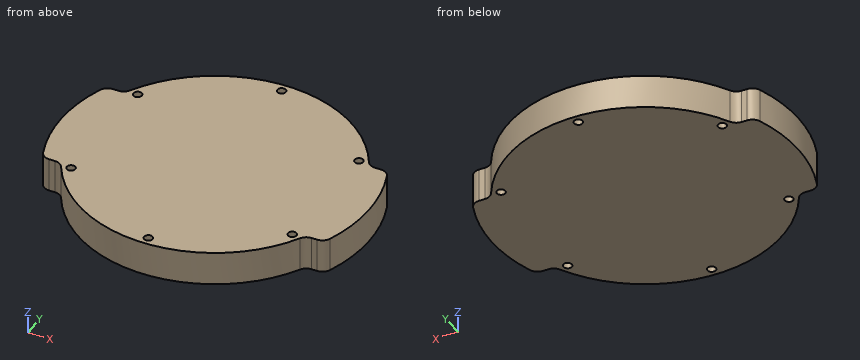
```python
from build123d import *

# Parameters (mm, degrees)
SKETCH_1_R          = 45.3
EXTRUDE_1_DEPTH     = 10
CUT_EXTRUDE_1_DEPTH = 11
FILLET_1_R          = 3
SKETCH_3_R          = 1.25
CUT_EXTRUDE_2_DEPTH = 11


with BuildPart() as part:
    # 草图1 → 凸台-拉伸1 (new body)
    with BuildSketch(Plane.XY):
        Circle(SKETCH_1_R)
    extrude(amount=EXTRUDE_1_DEPTH)

    # 草图2 → 切除-拉伸1 (cut, through all)
    with BuildSketch(Plane.XY.offset(10)):
        with BuildLine():
            Line((-36.056760808, 18), (-41.570301899, 18))
            ThreePointArc((-41.570301899, 18), (0, 45.3), (41.570301899, 18))
            Line((41.570301899, 18), (36.056760808, 18))
            ThreePointArc((36.056760808, 18), (0, 40.3), (-36.056760808, 18))
        make_face()
        with BuildLine():
            Line((-36.056760808, -18), (-41.734622438, -18))
            ThreePointArc((-41.734622438, -18), (0, -45.450838386), (41.734622438, -18))
            Line((41.734622438, -18), (36.056760808, -18))
            ThreePointArc((36.056760808, -18), (0, -40.3), (-36.056760808, -18))
        make_face()
    extrude(amount=-CUT_EXTRUDE_1_DEPTH, mode=Mode.SUBTRACT)

    # 圆角1
    fillet_1_edges = [part.edges().sort_by_distance(p)[0] for p in [
        (36.056760808, 18, 5),
        (-36.056760808, 18, 5),
        (-41.570301899, 18, 5),
        (41.570301899, 18, 5),
        (41.570301899, -18, 5),
        (36.056760808, -18, 5),
        (-41.570301899, -18, 5),
        (-36.056760808, -18, 5),
    ]]
    fillet(fillet_1_edges, radius=FILLET_1_R)

    # 草图3 → 切除-拉伸2 (cut, through all)
    with BuildSketch(Plane.XY.offset(10)):
        with Locations((0, 37.7)):
            Circle(SKETCH_3_R)
        with Locations((32.649157723, 18.85)):
            Circle(SKETCH_3_R)
        with Locations((32.649157723, -18.85)):
            Circle(SKETCH_3_R)
        with Locations((0, -37.7)):
            Circle(SKETCH_3_R)
        with Locations((-32.649157723, -18.85)):
            Circle(SKETCH_3_R)
        with Locations((-32.649157723, 18.85)):
            Circle(SKETCH_3_R)
    extrude(amount=-CUT_EXTRUDE_2_DEPTH, mode=Mode.SUBTRACT)


solid = part.part
```
Geometry check sheet. Reference: the model listing, model coordinates, mm. Give positions to 0.01 mm unless a question says otherwise; leave off trailing zeros. Write each loop counter-clockwise with the first axis right and the second up, starting at its lowest first coordinate (ties: lowest second). Pieces come first, ordered by that corner, then holes. Notation, with made-up numbers: (-34, 6) -> (-1, 6) arc R18 cw to (-1, 14) -> close; hole circle Ø3 at (47.5, -27). An arc over 180 degrees is marked (long way). Use one line per item in the form item = value.
Item 1: Depth check by flat-ended pin: pin 1 Ø5 at (y, z) = (31, 6.5) entering from -X; pin 2 Ø1.3 at (x, z) = (-39, 4.5) entering from -Y; pin 3 Ø0.8 at (x, z) = (-39, 2.5) entering from +Y. Enter the tip coordinate at first touch or a pass-through.
Results list:
pin_1 = -28.49
pin_2 = -18
pin_3 = 18
Item 2: Scan lines: line 1 (Y direction, x = 32, z = 1); line 2 (Y direction, x = 1, z = 4.5); line 3 (X direction, y = 18.5, z = 5). Record each from-to range of solid material in increasing order.
Results list:
line_1 = -24.5 to -19.92, -17.78 to 17.78, 19.92 to 24.5
line_2 = -40.29 to -38.45, -36.95 to 36.95, 38.45 to 40.29
line_3 = -36.21 to -33.85, -31.45 to 31.45, 33.85 to 36.21
Item 3: Sectioned sample at B-B on z = 3.75. Enter the section's corners in (x, y).
Results list:
outline = (-42.36, -16.06) arc R3 ccw to (-39.55, -18) -> (-37.87, -18) arc R3 cw to (-35.24, -19.55) arc R40.3 ccw to (35.24, -19.55) arc R3 cw to (37.87, -18) -> (39.55, -18) arc R3 ccw to (42.36, -16.06) arc R45.3 ccw to (42.36, 16.06) arc R3 ccw to (39.55, 18) -> (37.87, 18) arc R3 cw to (35.24, 19.55) arc R40.3 ccw to (-35.24, 19.55) arc R3 cw to (-37.87, 18) -> (-39.55, 18) arc R3 ccw to (-42.36, 16.06) arc R45.3 ccw to start; hole circle Ø2.5 at (-32.65, -18.85); hole circle Ø2.5 at (-32.65, 18.85); hole circle Ø2.5 at (0, -37.7); hole circle Ø2.5 at (0, 37.7); hole circle Ø2.5 at (32.65, -18.85); hole circle Ø2.5 at (32.65, 18.85)
Item 4: Sectioned sample at D-D on x = -23. Enter the section's corners in (y, z).
Results list:
outline = (-33.09, 0) -> (33.09, 0) -> (33.09, 10) -> (-33.09, 10) -> close
Item 5: Sectioned sample at C-C on y = 37.7. Enter the section's corners in (x, z), plus the area to 3 significant figures.
Results list:
outline = (-14.24, 0) -> (-1.25, 0) -> (-1.25, 10) -> (-14.24, 10) -> close; (1.25, 0) -> (14.24, 0) -> (14.24, 10) -> (1.25, 10) -> close
area = 260 mm2
Item 6: Sectioned sample at A-A on x = 0. Enter the section's corners in (y, z).
Results list:
outline = (-40.3, 0) -> (-38.95, 0) -> (-38.95, 10) -> (-40.3, 10) -> close; (-36.45, 0) -> (36.45, 0) -> (36.45, 10) -> (-36.45, 10) -> close; (38.95, 0) -> (40.3, 0) -> (40.3, 10) -> (38.95, 10) -> close
